Read the model definition and answer for the solid it produces. Units are mm, in the model's axes. Face numbers are marked on the shaded views. A direction names the side the tool comes from. Coordinates: 2 decimals unless noted, no trailing zeros. Write each loop counter-clockwise with the first axis right and the second up, starting at its lowest first coordinate (ties: lowest second). Pieces come first, ordered by that corner, then holes. Notation, with made-up numbers: (36, 6.5) - (48, 6.5) arc R20 cw to (48, 13.5) - close; hole circle Ø11 at (57, 9.25). An arc over 180 degrees is marked (long way). Return JSON: item names as keys, results as strings.
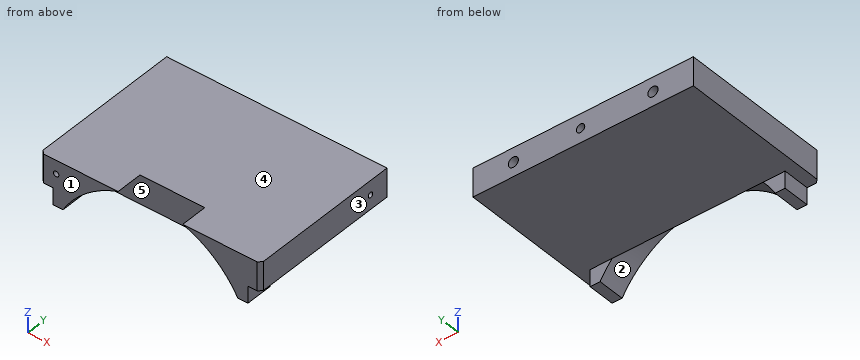
```python
from build123d import *

# Parameters (mm, degrees)
SKETCH1_W                 = 65.54
SKETCH1_H                 = 46
BOSS_EXTRUDE1_DEPTH       = 3.5
SKETCH2_W                 = 58
SKETCH2_H                 = 8
BOSS_EXTRUDE2_DEPTH       = 10
CUT_EXTRUDE1_DEPTH        = 8
BOSS_EXTRUDE3_DEPTH       = 5
CHAMFER1_SIZE             = 1
F_3_0MM_DOWEL_HOLE1_D     = 3
F_3_0MM_DOWEL_HOLE1_DEPTH = 4.5
F_3_0MM_DOWEL_HOLE1_TIP   = 0.901290929
M3X0_5_TAPPED_HOLE1_D     = 2.5
M3X0_5_TAPPED_HOLE1_DEPTH = 7.5
M3X0_5_TAPPED_HOLE1_TIP   = 0.751075774
M2X0_4_TAPPED_HOLE1_D     = 1.6
M2X0_4_TAPPED_HOLE1_DEPTH = 5.2
M2X0_4_TAPPED_HOLE1_TIP   = 0.480688495
M2X0_4_TAPPED_HOLE2_D     = 1.6
M2X0_4_TAPPED_HOLE2_DEPTH = 5.2
M2X0_4_TAPPED_HOLE2_TIP   = 0.480688495


with BuildPart() as part:
    # Sketch1 → Boss-Extrude1 (new body)
    with BuildSketch(Plane.XY):
        Rectangle(SKETCH1_W, SKETCH1_H)
    extrude(amount=BOSS_EXTRUDE1_DEPTH)

    # Sketch2 → Boss-Extrude2 (add)
    with BuildSketch(Plane(origin=(0, 0, 0), x_dir=(-1, 0, 0), z_dir=(0, 0, -1))):
        with Locations((0, -19)):
            Rectangle(SKETCH2_W, SKETCH2_H)
    extrude(amount=BOSS_EXTRUDE2_DEPTH)

    # Sketch5 → Cut-Extrude1 (cut)
    with BuildSketch(Plane.XZ.offset(23)):
        with BuildLine():
            Line((-26.311212976, -10.5), (26.311212976, -10.5))
            ThreePointArc((26.311212976, -10.5), (19.200628572, -1.861773381), (9.41946352, 3.570369836))
            Line((9.41946352, 3.570369836), (9.41946352, 4))
            Line((9.41946352, 4), (-9.622947545, 4))
            Line((-9.622947545, 4), (-9.622947545, 3.502268118))
            ThreePointArc((-9.622947545, 3.502268118), (-19.282941975, -1.930587904), (-26.311212976, -10.5))
        make_face()
    extrude(amount=-CUT_EXTRUDE1_DEPTH, mode=Mode.SUBTRACT)

    # Sketch6 → Boss-Extrude3 (add)
    with BuildSketch(Plane(origin=(0, 0, 0), x_dir=(-1, 0, 0), z_dir=(0, 0, -1))):
        Polygon((-32.77, 23), (-32.77, -23), (-29, -23), (-29, -15), (29, -15), (29, -23), (32.77, -23), (32.77, 23), align=None)
    extrude(amount=BOSS_EXTRUDE3_DEPTH)

    # Chamfer1
    chamfer1_edges = [part.edges().sort_by_distance(p)[0] for p in [
        (32.77, -23, -0.75),
        (-32.77, -23, -0.75),
    ]]
    chamfer(chamfer1_edges, length=CHAMFER1_SIZE)

    # Ø3.0mm Dowel Hole1
    with Locations(Plane(origin=(0, 23, 0), x_dir=(1, 0, 0), z_dir=(0, 1, 0))):
        with Locations((-20.77, 0.75), (20.77, 0.75)):
            Hole(F_3_0MM_DOWEL_HOLE1_D / 2, depth=F_3_0MM_DOWEL_HOLE1_DEPTH)
            with Locations((0, 0, -(F_3_0MM_DOWEL_HOLE1_DEPTH + F_3_0MM_DOWEL_HOLE1_TIP / 2))):  # 118° drill point
                Cone(0, F_3_0MM_DOWEL_HOLE1_D / 2, F_3_0MM_DOWEL_HOLE1_TIP, mode=Mode.SUBTRACT)

    # M3x0.5 Tapped Hole1
    with Locations(Plane(origin=(0, 23, 0), x_dir=(1, 0, 0), z_dir=(0, 1, 0))):
        with Locations((0.77, 0.75)):
            Hole(M3X0_5_TAPPED_HOLE1_D / 2, depth=M3X0_5_TAPPED_HOLE1_DEPTH)
            with Locations((0, 0, -(M3X0_5_TAPPED_HOLE1_DEPTH + M3X0_5_TAPPED_HOLE1_TIP / 2))):  # 118° drill point
                Cone(0, M3X0_5_TAPPED_HOLE1_D / 2, M3X0_5_TAPPED_HOLE1_TIP, mode=Mode.SUBTRACT)

    # M2x0.4 Tapped Hole1
    with Locations(Plane(origin=(0, -23, 0), x_dir=(-1, 0, 0), z_dir=(0, -1, 0))):
        with Locations((28.0334, 0.5)):
            Hole(M2X0_4_TAPPED_HOLE1_D / 2, depth=M2X0_4_TAPPED_HOLE1_DEPTH)
            with Locations((0, 0, -(M2X0_4_TAPPED_HOLE1_DEPTH + M2X0_4_TAPPED_HOLE1_TIP / 2))):  # 118° drill point
                Cone(0, M2X0_4_TAPPED_HOLE1_D / 2, M2X0_4_TAPPED_HOLE1_TIP, mode=Mode.SUBTRACT)

    # M2x0.4 Tapped Hole2
    with Locations(Plane(origin=(32.77, 0, 0), x_dir=(0, 0, -1), z_dir=(1, 0, 0))):
        with Locations((0.75, 17)):
            Hole(M2X0_4_TAPPED_HOLE2_D / 2, depth=M2X0_4_TAPPED_HOLE2_DEPTH)
            with Locations((0, 0, -(M2X0_4_TAPPED_HOLE2_DEPTH + M2X0_4_TAPPED_HOLE2_TIP / 2))):  # 118° drill point
                Cone(0, M2X0_4_TAPPED_HOLE2_D / 2, M2X0_4_TAPPED_HOLE2_TIP, mode=Mode.SUBTRACT)


solid = part.part
```
(1) Which of the six approach directions +Z, -Z, +X, -X, +Y, -Y give full straight-line access (tool end or side, diameter ignored) to the marked faces 1 and 2?
Answer:
{"face 1": "+Z, -Z, +X, -X, -Y", "face 2": "-Z, -Y"}
(2) Straight lines are drawn through the part: line 1 (Y direction, x = 30.9, z = -0.75); line 2 (Z direction, x = 20.77, y = 19.75); line 3 (Z direction, x = -14, y = 14). For each, find the intervals that lie inside material, in ascending order. Write a range as from..to.
Answer:
{"line 1": "-23..16.2, 17.8..23", "line 2": "-5..-2.25, 0.75..3.5", "line 3": "-5..3.5"}
(3) A cutting plane is placed at A-A (z = -5.75). Determine the outline of the cut face in (x, y).
Answer:
{"outline": "(-29, -23) - (-23.08, -23) - (-23.08, -15) - (-29, -15) - close; (23.08, -23) - (29, -23) - (29, -15) - (23.08, -15) - close"}
(4) A cutting plane is placed at B-B (y = -10). Determine the outline of the cut face in (x, z).
Answer:
{"outline": "(-32.77, -5) - (32.77, -5) - (32.77, 3.5) - (-32.77, 3.5) - close"}
(5) Determine the mould class of the marked faces 3, 4 and 5 for opening direction X: +X half, -X half, draft (parallel to the pull), parting line (faces both ways), or undercut.
Answer:
{"face 3": "+X half", "face 4": "draft", "face 5": "undercut"}
(6) Flat-ended cylindrical pins translate along their axes: P1, Ø1.5, axis at y = -18.5, z = -8.5, coming from the -X side; P2, Ø6, axis at x = -4.5, z = 1, coming from the -Y side; P3, Ø12, axis at x = -16.5, y = -2.5, coming from the -Z side. Find the tip coordinate at first contact, or state that the pin passes through.
Answer:
{"P1": "x = -29", "P2": "y = -15", "P3": "z = -5"}
(7) A cutting plane is placed at C-C (z = 2). Determine the outline of the cut face in (x, y), and give its area (3 significant figures).
Answer:
{"outline": "(-32.77, -22) - (-31.77, -23) - (-13.26, -23) - (-13.26, -15) - (13.26, -15) - (13.26, -23) - (31.77, -23) - (32.77, -22) - (32.77, 23) - (-32.77, 23) - close", "area": "2,800 mm²"}
